Read the model definition and answer for the solid it produces. Units are mm, in the model's axes. A direction names the side the tool comes from. Coordinates: 2 decimals unless noted, no trailing zeros. Write each loop counter-clockwise with the first axis right and the second up, starting at its lowest first coordinate (ties: lowest second). Pieces come first, ordered by that corner, then holes. Notation, with made-up numbers: M 60,66 L 82,66 A31 ccw 82,95 Z; hole C -9.75,23.25 d7. An arc over 180 degrees is marked long. Use a Markdown table: item, result. Add a question column.
from build123d import *

# Parameters (mm, degrees)
CROQUIS1_W              = 210
CROQUIS1_H              = 23
SALIENTE_EXTRUIR2_DEPTH = 23
REDONDEO4_R             = 23
CROQUIS2_W              = 23
CROQUIS2_H              = 23
SALIENTE_EXTRUIR3_DEPTH = 170
CROQUIS8_W              = 19
CROQUIS8_H              = 19
CORTAR_EXTRUIR2_DEPTH   = 80


with BuildPart() as part:
    # Croquis1 → Saliente-Extruir2 (new body)
    with BuildSketch(Plane.XY):
        Rectangle(CROQUIS1_W, CROQUIS1_H)
    extrude(amount=SALIENTE_EXTRUIR2_DEPTH)

    # Redondeo4
    redondeo4_edges = [part.edges().sort_by_distance(p)[0] for p in [
        (105, 0, 0),
    ]]
    fillet(redondeo4_edges, radius=REDONDEO4_R - 0.0001)  # a hair under: the kernel refuses the full size

    # Croquis2 → Saliente-Extruir3 (add)
    with BuildSketch(Plane.XY.offset(23)):
        with Locations((93.5, 0)):
            Rectangle(CROQUIS2_W, CROQUIS2_H)
    extrude(amount=SALIENTE_EXTRUIR3_DEPTH)

    # Croquis8 → Cortar-Extruir2 (cut)
    with BuildSketch(Plane.ZY.offset(105)):
        with Locations((11.435856313, 0)):
            Rectangle(CROQUIS8_W, CROQUIS8_H)
    extrude(amount=-CORTAR_EXTRUIR2_DEPTH, mode=Mode.SUBTRACT)


solid = part.part
Item 1: For faces 1 (the flat face through (82, 0, 107)), 2 (the flat face through (105, 0, 107)), 3 (the flat face through (-66, 0, 1.936)), determine the directions among +Z, -Z, +X, -X, +Y, -Y from which every point of the face is accessible in a straight line to the end or side of a thin tool.
Item 2: Find section C-C on z = 130. Give the vertices of the cut face in (x, y).
Item 3: Find section A-A on x = -38.5. Give the vertices of the cut face in (y, z).
Item 4: Find section D-D on x = 57.5. Give the vertices of the cut face in (y, z).
Item 5: Consider probe 1 along Z at (x, y) = (-75.5, 0); probe 2 along X at (y, z) = (-7.5, 153); probe 3 along Z at (x, y) = (79, -6). Determine where each line is inside the solid, lowest interval first.
Item 6: Each of these flat-tipped pins is pushed along its axis until it touches: pin 1 (8 mm diameter, centred on x = 73.5, y = 3.5, fed in from +Z); pin 2 (3 mm diameter, centred on y = 7.5, z = 94, fed in from -X); pin 3 (5.5 mm diameter, centred on y = 4, z = 9, fed in from -X). Where does it stop, or does it pass through?
Item 7: Determine the mould class of faces 4 (the flat face through (-25, 0, 11)), 5 (the flat face through (38, -11.5, 17)), 6 (the flat face through (-13, 0, 23)) for opening direction Y: pulls with the +Y half, pulls with the -Y half, needs draft (parallel to the pull), parting line crosses it, or undercut.
Item 8: Find section B-B on y = 1.25. Give the vertices of the cut face in (x, z).
Geometry says:
| question | item | result |
|---|---|---|
| 1 | face 1 | +Z, -X, +Y, -Y |
| 1 | face 2 | +Z, -Z, +X, +Y, -Y |
| 1 | face 3 | -X |
| 2 | outline | M 82,-11.5 L 105,-11.5 L 105,11.5 L 82,11.5 Z |
| 3 | outline | M -11.5,0 L 11.5,0 L 11.5,23 L -11.5,23 Z; hole M -9.5,1.94 L 9.5,1.94 L 9.5,20.94 L -9.5,20.94 Z |
| 4 | outline | M -11.5,0 L 11.5,0 L 11.5,23 L -11.5,23 Z |
| 5 | probe 1 | z = 0 to 1.94, 20.94 to 23 |
| 5 | probe 2 | x = 82 to 105 |
| 5 | probe 3 | z = 0 to 23 |
| 6 | pin 1 | stops at z = 23 |
| 6 | pin 2 | stops at x = 82 |
| 6 | pin 3 | stops at x = -25 |
| 7 | face 4 | undercut |
| 7 | face 5 | pulls with the -Y half |
| 7 | face 6 | needs draft |
| 8 | outline | M -105,0 L 82,0 A23 ccw 105,23 L 105,193 L 82,193 L 82,23 L -105,23 L -105,20.94 L -25,20.94 L -25,1.94 L -105,1.94 Z |
